Geometry: final body of the model. Coordinates: model frame, mm. Face numbers are marked on the shaded views. A direction names the side the tool comes from. Give positions to 0.01 mm unless a question says otherwise; leave off trailing zeros. Loops run counter-clockwise (first coordinate to the right, second up) from the corner with the lowest first, then second, coordinate; pieces in that order, holes last. Notation, with made-up numbers: (-14, 27) -> (44, 27) arc R25 ccw to (44, 47) -> close; hole circle Ø4 at (20.5, 78.5). An arc over 180 degrees is marked (long way). Answer in a Markdown table with one row per item. Add a question column.
1) Draft query along Z for the marked faces 1, 2 and 3. Return one class per face: +Z half, -Z half, draft (parallel to the pull), parting line (faces both ways), or undercut.
2) Section query A-A (z = 0). Return the cut outline in (x, y), plus the area to 3 significant figures.
3) Section query D-D (z = -7.5). Return the cut outline in (x, y) (3 decimals).
4) First-contact query: P1, Ø6, axis at x = 0, y = 53.975, coming from the -Z side. Flat tip, straight axial feed; report the tip coordinate or a pass-through.
5) Access query for the marked faces 4, 5 and 6. Directions: +Z, -Z, +X, -X, +Y, -Y. A direction counts if a zero-diameter tool reaches every point of the face in a straight line with its end or side. Return the directions, or none.
6) Section query B-B (x = 0). Return the cut outline in (y, z).
7) Section query C-C (y = 28.5). Return the cut outline in (x, z), plus the area to 3 significant figures.
8) Line query: line 1 (Y direction, x = 0, z = 5.75); line 2 (Y direction, x = -0.25, z = 7.25); line 3 (X direction, y = 29.5, z = 1). Output: solid intervals per line, ascending. Write a range as from..to.
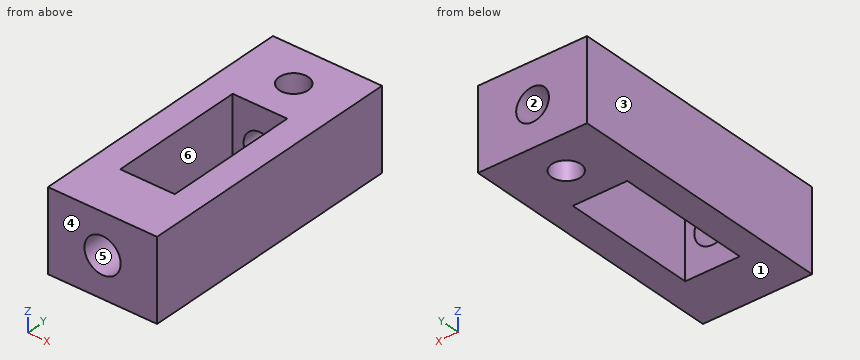
Autodesk Inventor part; units mm, degrees
ref_plane "YZ Plane" through (0, 0, 0) normal (1, 0, 0) x (0, 1, 0)
ref_plane "XZ Plane" through (0, 0, 0) normal (0, 1, 0) x (-1, 0, 0)
ref_plane "XY Plane" through (0, 0, 0) normal (0, 0, 1) x (1, 0, 0)
sketch "Sketch7" plane through (0, 0, 0) normal (0, 1, 0) x (-1, 0, 0)
  line L0 (12.7, 9.398) -> (-12.7, 9.398)
  line L1 (-12.7, 9.398) -> (-12.7, -9.398)
  line L2 (-12.7, -9.398) -> (12.7, -9.398)
  line L3 (12.7, -9.398) -> (12.7, 9.398)
  line L4 (12.7, 9.398) -> (-12.7, -9.398) construction
  line L5 (-12.7, 9.398) -> (12.7, -9.398) construction
  point P0 (0, 0)
  dimension "d53" = 18.796
  dimension "d54" = 25.4
extrude "Extrusion4" add sketch "Sketch7" along normal blind 63.5
sketch "Sketch8" plane through (0, 0, 0) normal (0, -1, 0) x (1, 0, 0)
  point P0 (0, 0)
  point P1 (0, 0)
hole "Hole7" at (0, 0, 0) direction (0, 1, 0) diameter 8.4328 depth 12.7
sketch "Sketch10" plane through (12.7, 0, -9.398) normal (0, 0, -1) x (-1, 0, 0)
  line L0 (25.4, 63.5) -> (0, 63.5) construction
  line L1 (12.7, 63.5) -> (12.7, 0) construction
  line L2 (25.4, 0) -> (0, 0) construction
  point P0 (12.7, 53.975)
  dimension "d77" = 9.525
hole "Hole8" at (0, 53.975, -9.398) direction (0, 0, 1) diameter 6.7564 end through all
sketch "Sketch11" plane through (-12.7, 0, 9.398) normal (0, 0, 1) x (1, 0, 0)
  line L0 (12.7, 0) -> (12.7, 63.5) construction
  line L1 (0, 63.5) -> (25.4, 63.5) construction
  line L2 (19.05, 12.7) -> (19.05, 44.45)
  line L3 (19.05, 44.45) -> (6.35, 44.45)
  line L4 (6.35, 44.45) -> (6.35, 12.7)
  line L5 (6.35, 12.7) -> (19.05, 12.7)
  line L6 (19.05, 12.7) -> (6.35, 44.45) construction
  line L7 (19.05, 44.45) -> (6.35, 12.7) construction
  line L8 (0, 0) -> (25.4, 0)
  point P0 (12.7, 28.575)
  dimension "d85" = 12.7
  dimension "d86" = 31.75
  dimension "d87" = 12.7
extrude "Extrusion5" cut sketch "Sketch11" against normal through all
sketch "Sketch12" plane through (0, 63.5, 0) normal (0, 1, 0) x (1, 0, 0)
  point P0 (0, 0)
  point P1 (0, 0)
hole "Hole9" at (0, 63.5, 0) direction (0, -1, 0) diameter 7.62 depth 19.05 tip angle 118
properties part number "BracketForEndOfDartActuator"
Evaluation:
| question | item | result |
|---|---|---|
| 1 | face 1 | -Z half |
| 1 | face 2 | undercut |
| 1 | face 3 | draft |
| 2 | outline | (-12.7, 0) -> (-4.22, 0) -> (-4.22, 12.7) -> (-6.35, 12.7) -> (-6.35, 44.45) -> (-3.81, 44.45) -> (-3.81, 63.5) -> (-12.7, 63.5) -> close; (3.81, 44.45) -> (6.35, 44.45) -> (6.35, 12.7) -> (4.22, 12.7) -> (4.22, 0) -> (12.7, 0) -> (12.7, 63.5) -> (3.81, 63.5) -> close |
| 2 | area | 957 mm² |
| 3 | outline | (-12.7, 0) -> (12.7, 0) -> (12.7, 63.5) -> (-12.7, 63.5) -> close; hole (-6.35, 12.7) -> (6.35, 12.7) -> (6.35, 44.45) -> (-6.35, 44.45) -> close; hole circle Ø6.756 at (0, 53.975) |
| 4 | P1 | through |
| 5 | face 4 | +Z, -Z, +X, -X, -Y |
| 5 | face 5 | -Y |
| 5 | face 6 | +Z, -Z |
| 6 | outline | (0, -9.4) -> (12.7, -9.4) -> (12.7, -4.22) -> (0, -4.22) -> close; (0, 4.22) -> (12.7, 4.22) -> (12.7, 9.4) -> (0, 9.4) -> close; (44.45, -9.4) -> (50.6, -9.4) -> (50.6, -3.81) -> (44.45, -3.81) -> close; (44.45, 3.81) -> (50.6, 3.81) -> (50.6, 9.4) -> (44.45, 9.4) -> close; (57.35, -9.4) -> (63.5, -9.4) -> (63.5, -3.81) -> (57.35, -3.81) -> close; (57.35, 3.81) -> (63.5, 3.81) -> (63.5, 9.4) -> (57.35, 9.4) -> close |
| 7 | outline | (-12.7, -9.4) -> (-6.35, -9.4) -> (-6.35, 9.4) -> (-12.7, 9.4) -> close; (6.35, -9.4) -> (12.7, -9.4) -> (12.7, 9.4) -> (6.35, 9.4) -> close |
| 7 | area | 239 mm² |
| 8 | line 1 | 0..12.7, 44.45..50.6, 57.35..63.5 |
| 8 | line 2 | 0..12.7, 44.45..50.61, 57.34..63.5 |
| 8 | line 3 | -12.7..-6.35, 6.35..12.7 |
